```python
from build123d import *

# Parameters (mm, degrees)
SKETCH1_W           = 29.591
SKETCH1_H           = 28.575
BOSS_EXTRUDE1_DEPTH = 3.175
BOSS_EXTRUDE2_DEPTH = 11.049
SKETCH3_W           = 18.796
SKETCH3_H           = 17.526
CUT_EXTRUDE1_DEPTH  = 3.175


with BuildPart() as part:
    # Sketch1 → Boss-Extrude1 (new body)
    with BuildSketch(Plane.XY):
        Rectangle(SKETCH1_W, SKETCH1_H)
    extrude(amount=BOSS_EXTRUDE1_DEPTH)

    # Sketch2 → Boss-Extrude2 (add, symmetric)
    with BuildSketch(Plane(origin=(0, 0, 0), x_dir=(0, 0, -1), z_dir=(1, 0, 0))):
        with BuildLine():
            Line((0, -14.2875), (11.684, -5.724576677))
            Line((11.684, -5.724576677), (11.684, -3.2385))
            Line((11.684, -3.2385), (6.0833, -3.2385))
            ThreePointArc((6.0833, -3.2385), (2.8448, 0), (6.0833, 3.2385))
            Line((6.0833, 3.2385), (11.684, 3.2385))
            Line((11.684, 3.2385), (11.684, 5.724576677))
            Line((11.684, 5.724576677), (0, 14.2875))
            Line((0, 14.2875), (0, -14.2875))
        make_face()
    extrude(amount=BOSS_EXTRUDE2_DEPTH, both=True)

    # Sketch3 → Cut-Extrude1 (cut)
    with BuildSketch(Plane.XY.offset(3.175)):
        Rectangle(SKETCH3_W, SKETCH3_H)
    extrude(amount=-CUT_EXTRUDE1_DEPTH, mode=Mode.SUBTRACT)


solid = part.part
```
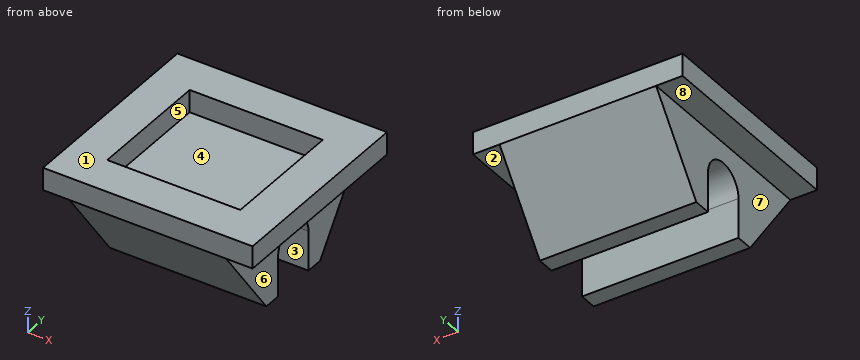
For this review, take the finished solid that the model builds, in its own axes (mm). Face numbers are marked on the shaded views. A direction names the side the tool comes from. Give positions to 0.01 mm unless a question says otherwise; leave off trailing zeros. Loops run counter-clockwise (first coordinate to the right, second up) from the corner with the lowest first, then second, coordinate; pieces in that order, holes last. Notation, with made-up numbers: M -4.5,16.25 L 42.5,16.25 A30 ccw 42.5,53.25 Z; hole C 7.25,51.25 d5. An arc over 180 degrees is marked long. One line per item, written item: value. Start each with the question number.
Q1. Clearance check with flat-ended pins moving along their axes: pin 1 Ø4.5 at (x, z) = (-3, -8) entering from +Y; pin 2 Ø6 at (y, z) = (5.5, -8.5) entering from +X; pin 3 Ø3 at (x, z) = (-5, -9.5) entering from -Y. State where each tip first meets the part, or that it passes through.
Q2. Machinability: for the marked faces 1, 2, 3 and 4, which of the approach directions +Z, -Z, +X, -X, +Y, -Y give a long, thin tool a straight path to every point of the face, cutting with its end or side? Answer none if there is none.
Q3. Add section B-B (z = -3.5). Give the boundary of the cut face in (x, y), and give its area (3 significant figures).
Q4. Add section A-A (y = 0). Give the boundary of the cut face in (x, z) (1 decimal), and give its area (3 significant figures).
Q5. Add section D-D (y = 3.75). Give the boundary of the cut face in (x, z) (1 decimal).
Q6. Add section C-C (x = -1.5). Give the boundary of the cut face in (y, z) (1 decimal).
Q7. For L1, parallel to X at y = 6.25, z = 2; L2, parallel to Y at x = -6.25, z = 1; L3, parallel to Z at x = 12.25, y = -3.25 (3 decimals), list the stretches that pass through material, from the lowest coordinate up.
Q8. Draft analysis for pull direction X (two halves, no side actions). For the marked faces 5, 6, 7 and 8, state which applies: released by +X, released by -X, zero draft, split by the parting line, or undercut.
Reply:
1. pin 1: y = 10.07
1. pin 2: x = 11.05
1. pin 3: y = -8.42
2. face 1: +Z, +X, -X, +Y, -Y
2. face 2: -Z, +X, +Y, -Y
2. face 3: -Z, +X, -X
2. face 4: +Z
3. outline: M -11.05,-11.72 L 11.05,-11.72 L 11.05,-1.95 L -11.05,-1.95 Z; M -11.05,1.95 L 11.05,1.95 L 11.05,11.72 L -11.05,11.72 Z
3. area: 432 mm²
4. outline: M -14.8,0 L -11,0 L -11,-2.8 L 11,-2.8 L 11,0 L 14.8,0 L 14.8,3.2 L 9.4,3.2 L 9.4,0 L -9.4,0 L -9.4,3.2 L -14.8,3.2 Z
4. area: 97.1 mm²
5. outline: M -14.8,0 L -11,0 L -11,-11.7 L 11,-11.7 L 11,0 L 14.8,0 L 14.8,3.2 L 9.4,3.2 L 9.4,0 L -9.4,0 L -9.4,3.2 L -14.8,3.2 Z
6. outline: M -14.3,0 L -5.7,-11.7 L -3.2,-11.7 L -3.2,-6.1 A3.2 cw 3.2,-6.1 L 3.2,-11.7 L 5.7,-11.7 L 14.3,0 L 14.3,3.2 L 8.8,3.2 L 8.8,0 L -8.8,0 L -8.8,3.2 L -14.3,3.2 Z
7. L1: -14.8 to -9.4, 9.4 to 14.8
7. L2: -14.29 to -8.76, 8.76 to 14.29
7. L3: 0 to 3.175
8. face 5: undercut
8. face 6: released by +X
8. face 7: released by -X
8. face 8: zero draft
